```python
from build123d import *

# Parameters (mm, degrees)
SKETCH21_R          = 16.15
SKETCH21_R_2        = 14.15
SKETCH25_R          = 14.15
SKETCH25_R_2        = 2
BOSS_EXTRUDE3_DEPTH = 2


with BuildPart() as part:
    # Sweep2: sweep along a path in Sketch1
    with BuildLine(Plane.XY) as sweep2_path:
        ThreePointArc((60.25, 0), (0, 60.25), (-60.25, 0))
    # Sketch21 → Sweep2 (sweep)
    with BuildSketch(Plane(origin=(60.25, 0, 0), x_dir=(1, 0, 0), z_dir=(0, 1, 0))):
        Circle(SKETCH21_R)
        Circle(SKETCH21_R_2, mode=Mode.SUBTRACT)
    sweep(path=sweep2_path.line)

    # Sketch25 → Boss-Extrude3 (add)
    with BuildSketch(Plane(origin=(-60.25, 0, 0), x_dir=(-1, 0, 0), z_dir=(0, -1, 0))):
        with BuildLine():
            Line((0, -16.15), (0, -24.183695576))
            Line((0, -24.183695576), (7.709659584, -24.183695576))
            Line((7.709659584, -24.183695576), (7.709659584, -14.190970689))
            ThreePointArc((7.709659584, -14.190970689), (16.15, 0), (7.709659584, 14.190970689))
            Line((7.709659584, 14.190970689), (7.709659584, 24.183695576))
            Line((7.709659584, 24.183695576), (0, 24.183695576))
            Line((0, 24.183695576), (0, 16.15))
            ThreePointArc((0, 16.15), (-16.15, 0), (0, -16.15))
        make_face()
        Circle(SKETCH25_R, mode=Mode.SUBTRACT)
        with Locations(Location((4, -20, 0), (0, 0, 180))):
            Circle(SKETCH25_R_2, mode=Mode.SUBTRACT)
        with Locations(Location((4, 20, 0), (0, 0, 180))):
            Circle(SKETCH25_R_2, mode=Mode.SUBTRACT)
    boss_extrude3 = extrude(amount=BOSS_EXTRUDE3_DEPTH)

    # Mirror3: Boss-Extrude3 across plane
    add(boss_extrude3.mirror(Plane(origin=(0, 0, 0), x_dir=(0, 0, 1), z_dir=(1, 0, 0))))


solid = part.part
```
Can you work these out from the model? Positions are in its coordinate system, mm. A direction names the side the tool comes from. Round coordinates to 2 decimals unless told otherwise and drop trailing zeros. Loops run counter-clockwise (first coordinate to the right, second up) from the corner with the lowest first, then second, coordinate; pieces in that order, holes last. Notation, with made-up numbers: (18.25, -23) -> (36.25, -23) arc R16 cw to (36.25, -17) -> close; hole circle Ø8 at (37, 57.25). An arc over 180 degrees is marked (long way). Answer in a Markdown table with one row per item.
Item 1: Suppose I cut it at A-A, the plane z = 20. List the corners of the cut face in (x, y) for me, plus the area to 3 significant figures.
Answer block:
| item | result |
|---|---|
| outline | (-67.96, -2) -> (-66.25, -2) -> (-66.25, 0) -> (-67.96, 0) -> close; (-62.25, -2) -> (-60.25, -2) -> (-60.25, 0) -> (-62.25, 0) -> close; (60.25, -2) -> (62.25, -2) -> (62.25, 0) -> (60.25, 0) -> close; (66.25, -2) -> (67.96, -2) -> (67.96, 0) -> (66.25, 0) -> close |
| area | 14.8 mm² |
Item 2: Will these pins go through, and if not, where does the flat tip stop? P1, Ø3.5, axis at x = -64.25, z = -20, coming from the +Y side; P2, Ø2, axis at y = -0.5, z = 20, coming from the +X side; P3, Ø3, axis at x = -24.5, z = -14.5, coming from the -Y side; P4, Ø0.6, axis at y = -1, z = 19, coming from the -X side.
Answer block:
| item | result |
|---|---|
| P1 | through |
| P2 | x = 67.96 |
| P3 | y = 44.21 |
| P4 | x = -67.96 |
Item 3: On a 3-axis mill with a long thin cutter (end or side, diameter ignored), from which of +Z, -Z, +X, -X, +Y, -Y can I reach the whole of each face in a straight line? I mean faces 5 (the flat face through (-62, 0, -19)), 6 (the cylindrical face through (46.114, -0.986, -0.622)), 7 (the flat face through (-75, -2, -2)). Say none if no direction works.
Answer block:
| item | result |
|---|---|
| face 5 | -Z, -X, +Y |
| face 6 | -Y |
| face 7 | +Z, -Z, +X, -X, -Y |
Item 4: If I drill on probe 1 along X at (y, z) = (-1.4, 0); probe 2 along X at (y, z) = (25, 7.5); probe 3 along Y at (x, z) = (-30, -4), over which ranges is the centre line in solid material (lowest first)?
Answer block:
| item | result |
|---|---|
| probe 1 | -76.4 to -74.4, -46.1 to -44.1, 44.1 to 46.1, 74.4 to 76.4 |
| probe 2 | -70.24 to -67.79, -41.27 to -38.55, 38.55 to 41.27, 67.79 to 70.24 |
| probe 3 | 33.01 to 35.76, 67.45 to 69.72 |
Item 5: We'd pull the mould along X, two halves only. Please class faces 1 (the cylindrical face through (76.4, -1, 0.2)), 2 (the cylindrical face through (-76.4, -1, 0.2)), 3 (the flat face through (62, 0, -19)), 4 (the cylindrical face through (64.51, -0.986, -18.017)): released by +X, released by -X, zero draft, split by the parting line, or undercut.
Answer block:
| item | result |
|---|---|
| face 1 | released by +X |
| face 2 | released by -X |
| face 3 | zero draft |
| face 4 | undercut |
Item 6: Suppose I cut it at B-B, the plane z = 11.5. List the corners of the cut face in (x, y) for me, plus the area to 3 significant figures.
Answer block:
| item | result |
|---|---|
| outline | (-71.59, -2) -> (-68.49, -2) -> (-68.49, 0) arc R68.49 cw to (68.49, 0) -> (68.49, -2) -> (71.59, -2) -> (71.59, 0) arc R71.59 ccw to (-71.59, 0) -> close; (-52.01, -2) -> (-48.91, -2) -> (-48.91, 0) arc R48.91 cw to (48.91, 0) -> (48.91, -2) -> (52.01, -2) -> (52.01, 0) arc R52.01 ccw to (-52.01, 0) -> close |
| area | 1,200 mm² |
Item 7: Suppose I cut it at C-C, the plane x = 64.25. Give the number of separate pieces and of enclosed holes in the cut face, plus the area to 3 significant figures.
Answer block:
| item | result |
|---|---|
| separate pieces | 3 |
| enclosed holes | 0 |
| area | 259 mm² |
